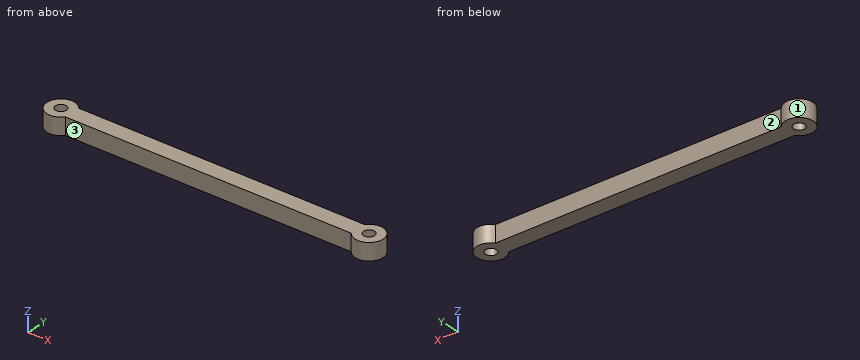
from build123d import *

# Parameters (mm, degrees)
SKETCH3_R           = 18.15695
SKETCH3_W           = 371.0727278
SKETCH3_H           = 21.9525
BOSS_EXTRUDE1_DEPTH = 10.97625
SKETCH4_R           = 7.1807
CUT_EXTRUDE1_DEPTH  = 645.139348927


with BuildPart() as part:
    # Sketch3 → Boss-Extrude1 (new, symmetric)
    with BuildSketch(Plane.XY):
        with Locations((-625.352112676, 0)):
            Circle(SKETCH3_R)
        with Locations((-225.352112676, 0)):
            Circle(SKETCH3_R)
        with Locations((-425.352112676, 0)):
            Rectangle(SKETCH3_W, SKETCH3_H)
    extrude(amount=BOSS_EXTRUDE1_DEPTH, both=True)

    # Sketch4 → Cut-Extrude1 (cut, through all)
    with BuildSketch(Plane.XY.offset(10.97625)):
        with Locations((-625.352112676, 0)):
            Circle(SKETCH4_R)
        with Locations((-225.352112676, 0)):
            Circle(SKETCH4_R)
    extrude(amount=-CUT_EXTRUDE1_DEPTH, mode=Mode.SUBTRACT)


solid = part.part
Build history of the part. All positions in model axes, mm. Face numbers are marked on the shaded views. A direction names the side the tool comes from. Coordinates: 2 decimals unless noted, no trailing zeros. Write each loop counter-clockwise with the first axis right and the second up, starting at its lowest first coordinate (ties: lowest second). Pieces come first, ordered by that corner, then holes.
(1) Cut at A-A on y = 0. List the corners of the cut face in (x, z).
(2) Cut at B-B on z = 1.75. List the corners of the cut face in (x, y), and give its area (3 significant figures).
(3) Cut at C-C on x = -366.5. List the corners of the cut face in (y, z).
(4) Pin check, flat tips, straight feed: pin 1 Ø6 at (x, z) = (-555.5, 2) entering from -Y; pin 2 Ø10 at (y, z) = (-10, -6) entering from -X; pin 3 Ø5 at (y, z) = (-9, -1.5) entering from +X. Stop position of each tip, or through.
(5) Drill centre lines: line 1 (X direction, y = -2, z = 9); line 2 (Y direction, x = -502, z = 9.5); line 3 (Y direction, x = -616.5, z = -0.5). Where is each one in solid material? Low to high.
(6) 3-axis set-ups, long thin cutter, end or side, ignore diameter. For the marked faces 1, 2 and 3: which of +Z, -Z, +X, -X, +Y, -Y reach the whole face in a straight line?
Working result:
1. outline: (-643.51, -10.98) - (-632.53, -10.98) - (-632.53, 10.98) - (-643.51, 10.98) - close; (-618.17, -10.98) - (-232.53, -10.98) - (-232.53, 10.98) - (-618.17, 10.98) - close; (-218.17, -10.98) - (-207.2, -10.98) - (-207.2, 10.98) - (-218.17, 10.98) - close
2. outline: (-610.89, -10.98) - (-239.82, -10.98) arc R18.16 ccw (long way) to (-239.82, 10.98) - (-610.89, 10.98) arc R18.16 ccw (long way) to start; hole circle Ø14.36 at (-625.35, 0); hole circle Ø14.36 at (-225.35, 0)
2. area: 9,780 mm2
3. outline: (-10.98, -10.98) - (10.98, -10.98) - (10.98, 10.98) - (-10.98, 10.98) - close
4. pin 1: stops at y = -10.98
4. pin 2: stops at x = -642.81
4. pin 3: stops at x = -208.4
5. line 1: x = -643.4 to -632.25, -618.46 to -232.25, -218.46 to -207.31
5. line 2: y = -10.98 to 10.98
5. line 3: y = -15.85 to 15.85
6. face 1: +Z, -Z
6. face 2: +Z, -Z, +Y
6. face 3: +Z, -Z, -Y
